Design review of the part shown in the three views and the two pictorial views. Dimensions are in mm from the part's minimum x, y and z. A direction names the side the tool comes from. Give positions to 0.01 mm unless a question says otherwise; leave off trailing zeros. Loops run counter-clockwise (first coordinate to the right, second up) from the corner with the lowest first, then second, coordinate; pieces in that order, holes last.
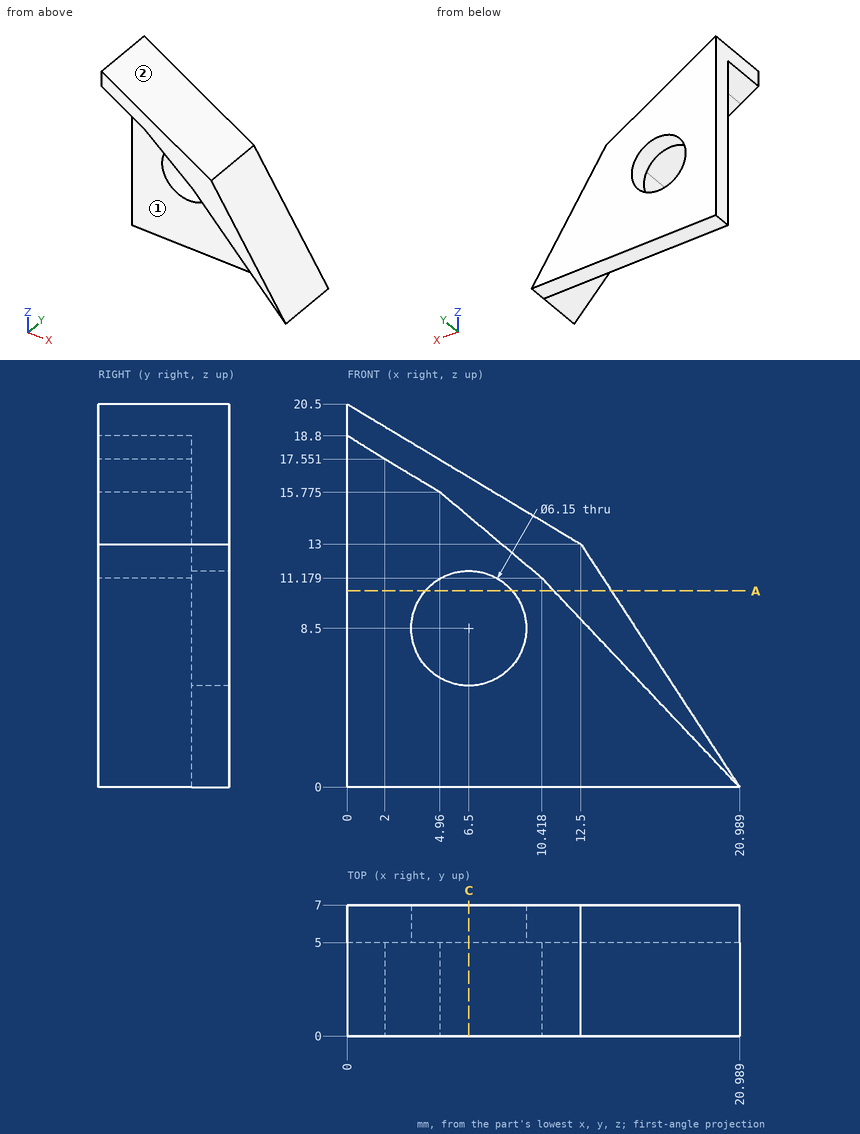
Q1. Take a section at A-A (z = 10.5). Give the boundary of the cut face in (x, y) (1 decimal).
Results:
outline: (0, 5) - (4.2, 5) - (4.2, 7) - (0, 7) - close; (8.8, 5) - (11.1, 5) - (11.1, 0) - (14.1, 0) - (14.1, 7) - (8.8, 7) - close
Q2. Insertion check: pin 1 (1.5 mm diameter, centred on y = 1, z = 8, fed in from +X) (1 decimal); pin 2 (2 mm diameter, centred on y = 2.5, z = 15, fed in from +X) (1 decimal); pin 3 (1.5 mm diameter, centred on y = 1.5, z = 4.5, fed in from +X). Each pin has a flat end and moves straight along its axis. Give the tip position at first contact, or say it passes through.
Results:
pin 1: stops at x = 16.3
pin 2: stops at x = 10.8
pin 3: stops at x = 18.54
Q3. Tool access review of the marked faces 1 and 2: name each direction out of +Z, -Z, +X, -X, +Y, -Y from which nothing blocks a thin tool from reaching the whole face with its end or side.
Results:
face 1: -Z, -X, -Y
face 2: +Z, +X, +Y, -Y
Q4. Wall thickness on line 1 (Y direction, x = 6, z = 13.75); line 2 (X direction, y = 5.5, z = 8.5) (1 decimal); line 3 (Z direction, x = 9, y = 6): over which ranges is each line inside the solid? List them lowest first.
Results:
line 1: y = 5 to 7
line 2: x = 0 to 3.4, 9.6 to 15.4
line 3: z = 0 to 6.71, 10.29 to 15.1
Q5. Take a section at C-C (x = 6.5). Give the boundary of the cut face in (y, z) (1 decimal).
Results:
outline: (0, 14.5) - (5, 14.5) - (5, 11.6) - (7, 11.6) - (7, 16.6) - (0, 16.6) - close; (5, 0) - (7, 0) - (7, 5.4) - (5, 5.4) - close
